```python
from build123d import *

# Parameters (mm, degrees)
SKETCH_1_W             = 268
SKETCH_1_H             = 38
EXTRUDE_1_DEPTH        = 278
SKETCH_2_W             = 260
SKETCH_2_H             = 270
CUT_EXTRUDE_1_DEPTH    = 36
CUT_EXTRUDE_2_REACH    = 311.194
SKETCH_3_W             = 100
SKETCH_3_H             = 16
FILLET_1_R             = 2
SKETCH_4_W             = 2
SKETCH_4_H             = 270
EXTRUDE_2_DEPTH        = 36
PATTERN_LINEAR_1_COUNT = 3
PATTERN_LINEAR_1_PITCH = 66
SKETCH_5_W             = 260
SKETCH_5_H             = 2
EXTRUDE_3_DEPTH        = 36
CUT_EXTRUDE_4_DEPTH    = 2
FILLET_2_R             = 2
PATTERN_LINEAR_2_COUNT = 3
PATTERN_LINEAR_2_PITCH = 70


with BuildPart() as part:
    # 草图1 → 凸台-拉伸1 (new body)
    with BuildSketch(Plane(origin=(0, 0, 0), x_dir=(1, 0, 0), z_dir=(0, 1, 0))):
        Rectangle(SKETCH_1_W, SKETCH_1_H)
    extrude(amount=EXTRUDE_1_DEPTH)

    # 草图2 → 切除-拉伸1 (cut)
    with BuildSketch(Plane(origin=(0, 0, -19), x_dir=(-1, 0, 0), z_dir=(0, 0, -1))):
        with Locations((0, 139)):
            Rectangle(SKETCH_2_W, SKETCH_2_H)
    extrude(amount=-CUT_EXTRUDE_1_DEPTH, mode=Mode.SUBTRACT)

    # 草图3 → 切除-拉伸2 (cut, up to next)
    with BuildSketch(Plane(origin=(0, 278, 0), x_dir=(1, 0, 0), z_dir=(0, 1, 0)), mode=Mode.PRIVATE) as cut_extrude_2_sk1:
        with Locations((0, 11)):
            Rectangle(SKETCH_3_W, SKETCH_3_H)
    cut_extrude_2_tool1 = extrude(cut_extrude_2_sk1.sketch, amount=-CUT_EXTRUDE_2_REACH, mode=Mode.PRIVATE) & part.part
    add(cut_extrude_2_tool1.solids().sort_by_distance((0, 278, -11))[0], mode=Mode.SUBTRACT)

    # 圆角1
    fillet_1_edges = [part.edges().sort_by_distance(p)[0] for p in [
        (134, 278, 0),
        (-50, 276, -3),
        (-50, 276, -19),
        (50, 276, -19),
        (50, 276, -3),
        (-134, 278, 0),
        (0, 0, -19),
        (134, 0, 0),
        (0, 0, 19),
        (-134, 0, 0),
        (-134, 139, -19),
        (134, 139, -19),
        (134, 139, 19),
        (-134, 139, 19),
    ]]
    fillet(fillet_1_edges, radius=FILLET_1_R)

    # 草图4 → 凸台-拉伸2 (add)
    with BuildSketch(Plane(origin=(0, 0, 17), x_dir=(-1, 0, 0), z_dir=(0, 0, -1))):
        with Locations((-67, 139)):
            Rectangle(SKETCH_4_W, SKETCH_4_H)
    extrude_2 = extrude(amount=EXTRUDE_2_DEPTH)

    # 阵列(线性)1: 凸台-拉伸2 ×3
    with Locations(*[(-i * PATTERN_LINEAR_1_PITCH, 0, 0) for i in range(1, PATTERN_LINEAR_1_COUNT)]):
        add(extrude_2)

    # 草图5 → 凸台-拉伸3 (add)
    with BuildSketch(Plane(origin=(0, 0, 17), x_dir=(-1, 0, 0), z_dir=(0, 0, -1))):
        with Locations((0, 209)):
            Rectangle(SKETCH_5_W, SKETCH_5_H)
    extrude_3 = extrude(amount=EXTRUDE_3_DEPTH)

    # 草图7 → 切除-拉伸4 (cut)
    with BuildSketch(Plane.ZY):
        with BuildLine():
            Line((-19, 274), (-19, 258))
            ThreePointArc((-19, 258), (-7.686291501, 262.686291501), (-3, 274))
            Line((-3, 274), (-19, 274))
        make_face()
    extrude(amount=-CUT_EXTRUDE_4_DEPTH, mode=Mode.SUBTRACT)

    # 圆角2
    fillet_2_edges = [part.edges().sort_by_distance(p)[0] for p in [
        (1, 258, -19),
    ]]
    fillet(fillet_2_edges, radius=FILLET_2_R)

    # 阵列(线性)2: 凸台-拉伸3 ×3
    with Locations(*[(0, -i * PATTERN_LINEAR_2_PITCH, 0) for i in range(1, PATTERN_LINEAR_2_COUNT)]):
        add(extrude_3)


solid = part.part
```
Design review of the part built by this model. Coordinates are the model's own, in mm. Give positions to 0.01 mm unless a question says otherwise; leave off trailing zeros. Write each loop counter-clockwise with the first axis right and the second up, starting at its lowest first coordinate (ties: lowest second). Pieces come first, ordered by that corner, then holes. Notation, with made-up numbers: (9, 88.5) -> (31, 88.5) arc R14 cw to (31, 99.5) -> close; hole circle Ø7 at (41, -38). An arc over 180 degrees is marked (long way). Answer in a Markdown table with one row per item.
(1) Consider section B-B (x = 42). State the section outline as (y, z) points, then the cut area to 3 significant figures.
Results:
| item | result |
|---|---|
| outline | (0, -17) arc R2 ccw to (2, -19) -> (4, -19) -> (4, 17) -> (68, 17) -> (68, -19) -> (70, -19) -> (70, 17) -> (138, 17) -> (138, -19) -> (140, -19) -> (140, 17) -> (208, 17) -> (208, -19) -> (210, -19) -> (210, 17) -> (274, 17) -> (274, -3) -> (278, -3) -> (278, 19) -> (2, 19) arc R2 ccw to (0, 17) -> close |
| area | 994 mm2 |
(2) Consider section C-C (z = 11.5). Count the separate pieces of the cut face and the enclosed holes in it, then the cut area to 3 significant figures.
Results:
| item | result |
|---|---|
| separate pieces | 1 |
| enclosed holes | 16 |
| area | 7,440 mm2 |
(3) Clearance check with a flat-ended pin moving along its axis: pin 1 (18.5 mm diameter, centred on x = 86, y = 112, fed in from -Z). State where the tip first meets the part, or that it passes through.
Results:
| item | result |
|---|---|
| pin 1 | z = 17 |
(4) Consider section D-D (x = -99). State the section outline as (y, z) points, then the cut area to 3 significant figures.
Results:
| item | result |
|---|---|
| outline | (0, -17) arc R2 ccw to (2, -19) -> (4, -19) -> (4, 17) -> (68, 17) -> (68, -19) -> (70, -19) -> (70, 17) -> (138, 17) -> (138, -19) -> (140, -19) -> (140, 17) -> (208, 17) -> (208, -19) -> (210, -19) -> (210, 17) -> (274, 17) -> (274, -19) -> (278, -19) -> (278, 19) -> (2, 19) arc R2 ccw to (0, 17) -> close |
| area | 1,060 mm2 |
(5) To check wall thickness, follow probe 1 along X at (y, z) = (160, 8); probe 2 along Y at (x, z) = (-76.5, 4); probe 3 along Y at (x, z) = (-27, -12). State the ranges of each line that lie inside material, in increasing order.
Results:
| item | result |
|---|---|
| probe 1 | -134 to -130, -66 to -64, 0 to 2, 66 to 68, 130 to 134 |
| probe 2 | 0 to 4, 68 to 70, 138 to 140, 208 to 210, 274 to 278 |
| probe 3 | 0 to 4, 68 to 70, 138 to 140, 208 to 210 |
(6) Consider section A-A (y = 58.5). State the section outline as (x, z) points, then the cut area to 3 significant figures.
Results:
| item | result |
|---|---|
| outline | (-134, -17) arc R2 ccw to (-132, -19) -> (-130, -19) -> (-130, 17) -> (-66, 17) -> (-66, -19) -> (-64, -19) -> (-64, 17) -> (0, 17) -> (0, -19) -> (2, -19) -> (2, 17) -> (66, 17) -> (66, -19) -> (68, -19) -> (68, 17) -> (130, 17) -> (130, -19) -> (132, -19) arc R2 ccw to (134, -17) -> (134, 17) arc R2 ccw to (132, 19) -> (-132, 19) arc R2 ccw to (-134, 17) -> close |
| area | 1,040 mm2 |
(7) Mouldability with a two-part tool opening along Y and no side actions: class faces 1 (the flat face through (-98, 208, -1)), 2 (the flat face through (0, 242, -1)), 3 (the flat face through (-2, 278, 0)), 4 (the flat face through (-2, 0, 0)) as +Y half, -Y half, draft (parallel to the pull), parting line (faces both ways), or undercut.
Results:
| item | result |
|---|---|
| face 1 | undercut |
| face 2 | undercut |
| face 3 | +Y half |
| face 4 | -Y half |
